Could you check a few things on this model? Use its own coordinates, in mm. A direction names the side the tool comes from. Coordinates: 2 decimals unless noted, no trailing zeros. Write each loop counter-clockwise with the first axis right and the second up, starting at its lowest first coordinate (ties: lowest second). Pieces come first, ordered by that corner, then holes.
```python
from build123d import *
from build123d.topology import SkipClean

# Parameters (mm, degrees)
BOSS_EXTRUDE1_DEPTH = 16
SKETCH3_R           = 3.75
CUT_EXTRUDE1_DEPTH  = 16
SKETCH4_R           = 8
SKETCH4_R_2         = 3.75
BOSS_EXTRUDE2_DEPTH = 16
BOSS_EXTRUDE3_START = 4
SKETCH5_R           = 3.75
BOSS_EXTRUDE3_DEPTH = 4
SKETCH6_R           = 8
SKETCH6_R_2         = 3.75
BOSS_EXTRUDE4_DEPTH = 16
SKETCH7_R           = 3.75
CUT_EXTRUDE2_DEPTH  = 16
BOSS_EXTRUDE5_START = 4
SKETCH8_R           = 3.75
BOSS_EXTRUDE5_DEPTH = 4


with BuildPart() as part:
    # Sketch1 → Boss-Extrude1 (new body)
    with BuildSketch(Plane.XY):
        Polygon((81.771892596, 8.5), (83.771892596, 8.5), (84.681818182, 6), (102.681818182, 6), (102.681818182, -6), (-75.13803299, -6), (-75.13803299, 6), (-57.13803299, 6), (-56.228107404, 8.5), (-54.228107404, 8.5), (-53.318181818, 6), (-51.13803299, 6), (-50.228107404, 8.5), (-48.228107404, 8.5), (-47.318181818, 6), (-45.13803299, 6), (-44.228107404, 8.5), (-42.228107404, 8.5), (-41.318181818, 6), (-39.13803299, 6), (-38.228107404, 8.5), (-36.228107404, 8.5), (-35.318181818, 6), (-33.13803299, 6), (-32.228107404, 8.5), (-30.228107404, 8.5), (-29.318181818, 6), (-27.13803299, 6), (-26.228107404, 8.5), (-24.228107404, 8.5), (-23.318181818, 6), (-21.13803299, 6), (-20.228107404, 8.5), (-18.228107404, 8.5), (-17.318181818, 6), (-15.13803299, 6), (-14.228107404, 8.5), (-12.228107404, 8.5), (-11.318181818, 6), (-9.13803299, 6), (-8.228107404, 8.5), (-6.228107404, 8.5), (-5.318181818, 6), (-3.13803299, 6), (-2.228107404, 8.5), (-0.228107404, 8.5), (0.681818182, 6), (2.86196701, 6), (3.771892596, 8.5), (5.771892596, 8.5), (6.681818182, 6), (8.86196701, 6), (9.771892596, 8.5), (11.771892596, 8.5), (12.681818182, 6), (14.86196701, 6), (15.771892596, 8.5), (17.771892596, 8.5), (18.681818182, 6), (20.86196701, 6), (21.771892596, 8.5), (23.771892596, 8.5), (24.681818182, 6), (26.86196701, 6), (27.771892596, 8.5), (29.771892596, 8.5), (30.681818182, 6), (32.86196701, 6), (33.771892596, 8.5), (35.771892596, 8.5), (36.681818182, 6), (38.86196701, 6), (39.771892596, 8.5), (41.771892596, 8.5), (42.681818182, 6), (44.86196701, 6), (45.771892596, 8.5), (47.771892596, 8.5), (48.681818182, 6), (50.86196701, 6), (51.771892596, 8.5), (53.771892596, 8.5), (54.681818182, 6), (56.86196701, 6), (57.771892596, 8.5), (59.771892596, 8.5), (60.681818182, 6), (62.86196701, 6), (63.771892596, 8.5), (65.771892596, 8.5), (66.681818182, 6), (68.86196701, 6), (69.771892596, 8.5), (71.771892596, 8.5), (72.681818182, 6), (74.86196701, 6), (75.771892596, 8.5), (77.771892596, 8.5), (78.681818182, 6), (80.86196701, 6), align=None)
    extrude(amount=BOSS_EXTRUDE1_DEPTH)

    # Sketch3 → Cut-Extrude1 (cut)
    with BuildSketch(Plane(origin=(0, 6, 0), x_dir=(1, 0, 0), z_dir=(0, 1, 0))):
        with BuildLine():
            Line((104.42249812, 2.008331966), (94.86196701, 0))
            Line((94.86196701, 0), (102.681818182, 0))
            Line((102.681818182, 0), (102.681818182, -6.311827124))
            ThreePointArc((102.681818182, -6.311827124), (102.816802313, -7.151121143), (102.86196701, -8))
            ThreePointArc((102.86196701, -8), (102.816802313, -8.848878857), (102.681818182, -9.688172876))
            Line((102.681818182, -9.688172876), (102.681818182, -16))
            Line((102.681818182, -16), (94.86196701, -16))
            Line((94.86196701, -16), (91.310905943, -17.982667731))
            Line((91.310905943, -17.982667731), (106.371238817, -17.331958931))
            Line((106.371238817, -17.331958931), (104.42249812, 2.008331966))
        make_face()
        with BuildLine():
            Line((102.681818182, 0), (94.86196701, 0))
            ThreePointArc((94.86196701, 0), (99.886636999, -1.774834018), (102.681818182, -6.311827124))
            Line((102.681818182, -6.311827124), (102.681818182, 0))
        make_face()
        with BuildLine():
            ThreePointArc((102.681818182, -9.688172876), (99.886636999, -14.225165982), (94.86196701, -16))
            Line((94.86196701, -16), (102.681818182, -16))
            Line((102.681818182, -16), (102.681818182, -9.688172876))
        make_face()
        with Locations(Location((94.86196701, -8, 0), (0, 0, 180))):
            Circle(SKETCH3_R)
    extrude(amount=-CUT_EXTRUDE1_DEPTH, mode=Mode.SUBTRACT)

    # Sketch4 → Boss-Extrude2 (add)
    with SkipClean():  # the faces are left unmerged after this step: merging them gives an invalid solid
        with BuildSketch(Plane(origin=(0, 6, 0), x_dir=(1, 0, 0), z_dir=(0, 1, 0))):
            with Locations(Location((94.86196701, -8, 0), (0, 0, 180))):
                Circle(SKETCH4_R)
            with Locations(Location((94.86196701, -8, 0), (0, 0, 180))):
                Circle(SKETCH4_R_2, mode=Mode.SUBTRACT)
        extrude(amount=-BOSS_EXTRUDE2_DEPTH)

    # Sketch5 → Boss-Extrude3 (add)
    with SkipClean():  # the faces are left unmerged after this step: merging them gives an invalid solid
        with BuildSketch(Plane(origin=(0, 6, 0), x_dir=(1, 0, 0), z_dir=(0, 1, 0)).offset(BOSS_EXTRUDE3_START)):
            with BuildLine():
                ThreePointArc((94.86196701, 0), (86.86196701, -8), (94.86196701, -16))
                ThreePointArc((94.86196701, -16), (100.51882126, -13.656854249), (102.86196701, -8))
                ThreePointArc((102.86196701, -8), (100.51882126, -2.343145751), (94.86196701, 0))
            make_face()
            with Locations(Location((94.86196701, -8, 0), (0, 0, 180))):
                Circle(SKETCH5_R, mode=Mode.SUBTRACT)
        extrude(amount=-BOSS_EXTRUDE3_DEPTH)

    # Sketch6 → Boss-Extrude4 (add)
    with SkipClean():  # the faces are left unmerged after this step: merging them gives an invalid solid
        with BuildSketch(Plane(origin=(0, 6, 0), x_dir=(1, 0, 0), z_dir=(0, 1, 0))):
            with Locations(Location((-67.318181818, -8, 0), (0, 0, 180))):
                Circle(SKETCH6_R)
            with Locations(Location((-67.318181818, -8, 0), (0, 0, 180))):
                Circle(SKETCH6_R_2, mode=Mode.SUBTRACT)
        extrude(amount=-BOSS_EXTRUDE4_DEPTH)

    # Sketch7 → Cut-Extrude2 (cut)
    with SkipClean():  # the faces are left unmerged after this step: merging them gives an invalid solid
        with BuildSketch(Plane(origin=(0, 6, 0), x_dir=(1, 0, 0), z_dir=(0, 1, 0))):
            with BuildLine():
                Line((-67.318181818, 0), (-75.13803299, 0))
                Line((-75.13803299, 0), (-75.13803299, -6.311827124))
                ThreePointArc((-75.13803299, -6.311827124), (-72.342851807, -1.774834018), (-67.318181818, 0))
            make_face()
            with BuildLine():
                ThreePointArc((-67.318181818, -16), (-72.342851807, -14.225165982), (-75.13803299, -9.688172876))
                Line((-75.13803299, -9.688172876), (-75.13803299, -16))
                Line((-75.13803299, -16), (-67.318181818, -16))
            make_face()
            with Locations(Location((-67.318181818, -8, 0), (0, 0, 180))):
                Circle(SKETCH7_R)
        extrude(amount=-CUT_EXTRUDE2_DEPTH, mode=Mode.SUBTRACT)
    add(part.part.scale(1), mode=Mode.REPLACE)  # the faces are merged on a copy

    # Sketch8 → Boss-Extrude5 (add)
    with SkipClean():  # the faces are left unmerged after this step: merging them gives an invalid solid
        with BuildSketch(Plane(origin=(0, 6, 0), x_dir=(1, 0, 0), z_dir=(0, 1, 0)).offset(BOSS_EXTRUDE5_START)):
            with BuildLine():
                ThreePointArc((-59.318181818, -8), (-61.661327569, -2.343145751), (-67.318181818, 0))
                ThreePointArc((-67.318181818, 0), (-75.318181818, -8), (-67.318181818, -16))
                ThreePointArc((-67.318181818, -16), (-61.661327569, -13.656854249), (-59.318181818, -8))
            make_face()
            with Locations(Location((-67.318181818, -8, 0), (0, 0, 180))):
                Circle(SKETCH8_R, mode=Mode.SUBTRACT)
        extrude(amount=-BOSS_EXTRUDE5_DEPTH)


solid = part.part
```
1. On a 3-axis mill with a long thin cutter (end or side, diameter ignored), from which of +Z, -Z, +X, -X, +Y, -Y can I reach the whole of each face in a straight line? I mean faces 1 (the face through (86, 6, 8)), 2 (the face through (-71, -10, 6)). Say none if no direction works.
Verdict:
face 1: +Y
face 2: +Z, -Z, +X, -X, -Y
2. Please list where these lines run through material, in increasing order: line 1 along X through (y, z) = (-4.5, 9.25); line 2 along X through (y, z) = (4.75, 5); line 3 along Y through (x, z) = (-40.5, 10.25).
Verdict:
line 1: x = -75.22 to -70.85, -63.78 to 91.33, 98.4 to 102.76
line 2: x = -74.73 to -69.57, -65.07 to 92.61, 97.11 to 102.28
line 3: y = -6 to 6
3. For pin 1 (3 mm diameter, centred on x = 43, z = 6, fed in from +Y); pin 2 (1 mm diameter, centred on y = 0, z = 12.5, fed in from -X); pin 3 (1.1 mm diameter, centred on x = -52, z = 9.5, fed in from +Y); pin 4 (6 mm diameter, centred on x = 72.5, y = 8, fed in from -Z), each with a flat end and sliding along its axis, tell me the tip position at first contact or that it passes through.
Verdict:
pin 1: stops at y = 8.5
pin 2: stops at x = -74.25
pin 3: stops at y = 6
pin 4: stops at z = 0
4. I want a section at A-A on y = -0.75. Please give me the cut outline in (x, z).
Verdict:
outline: (-67.32, 0) - (94.86, 0) arc R8 ccw to (94.86, 16) - (-67.32, 16) arc R8 ccw to start; hole circle Ø7.5 at (-67.32, 8); hole circle Ø7.5 at (94.86, 8)
5. If we mould it in two halves opening along Z, with no side actions, what happens to faces 3 (the face through (15, 0, 16)), 4 (the face through (98.3, 10, 6.1)), 5 (the face through (-63.57, 0.14, 8.16))? For each: pulls with the +Z half, pulls with the -Z half, needs draft (parallel to the pull), parting line crosses it, or undercut.
Verdict:
face 3: pulls with the +Z half
face 4: needs draft
face 5: undercut
